```python
from build123d import *

# Parameters (mm, degrees)
SKETCH1_W           = 110
SKETCH1_H           = 30
BOSS_EXTRUDE1_DEPTH = 12
FILLET1_R           = 10
FILLET2_R           = 10
SKETCH9_R           = 12
CUT_EXTRUDE5_DEPTH  = 11
SKETCH13_R          = 12
CUT_EXTRUDE7_DEPTH  = 11
SKETCH15_R          = 3.43
SKETCH15_R_2        = 1
CUT_EXTRUDE8_DEPTH  = 123.394479271
SKETCH16_R          = 3.43
SKETCH16_R_2        = 1
CUT_EXTRUDE9_DEPTH  = 123.394479271


with BuildPart() as part:
    # Sketch1 → Boss-Extrude1 (new body)
    with BuildSketch(Plane(origin=(0, 0, 0), x_dir=(1, 0, 0), z_dir=(0, 1, 0))):
        with Locations((5.385430756, 3.53837453)):
            Rectangle(SKETCH1_W, SKETCH1_H)
    extrude(amount=BOSS_EXTRUDE1_DEPTH)

    # Fillet1
    fillet1_edges = [part.edges().sort_by_distance(p)[0] for p in [
        (-49.614569244, 6, -18.53837453),
        (-49.614569244, 6, 11.46162547),
    ]]
    fillet(fillet1_edges, radius=FILLET1_R)

    # Fillet2
    fillet2_edges = [part.edges().sort_by_distance(p)[0] for p in [
        (60.385430756, 6, -18.53837453),
        (60.385430756, 6, 11.46162547),
    ]]
    fillet(fillet2_edges, radius=FILLET2_R)

    # Sketch9 → Cut-Extrude5 (cut)
    with BuildSketch(Plane(origin=(0, 12, 0), x_dir=(1, 0, 0), z_dir=(0, 1, 0))):
        with Locations(Location((-31.195762423, 3.53837453, 0), (0, 0, 270))):
            Circle(SKETCH9_R)
    extrude(amount=-CUT_EXTRUDE5_DEPTH, mode=Mode.SUBTRACT)

    # Sketch13 → Cut-Extrude7 (cut)
    with BuildSketch(Plane(origin=(70.696833098, 12, 1.072209922), x_dir=(1, 0, 0), z_dir=(0, 1, 0))):
        with Locations(Location((-31.195762423, 3.53837453, 0), (0, 0, 270))):
            Circle(SKETCH13_R)
    extrude(amount=-CUT_EXTRUDE7_DEPTH, mode=Mode.SUBTRACT)

    # Sketch15 → Cut-Extrude8 (cut, through all)
    with BuildSketch(Plane(origin=(70.696833098, 1, 1.072209922), x_dir=(1, 0, 0), z_dir=(0, 1, 0))):
        with Locations(Location((-31.147671482, 3.53837453, 0), (0, 0, 270))):
            Circle(SKETCH15_R)
        with Locations(Location((-25.217671482, 3.53837453, 0), (0, 0, 270))):
            Circle(SKETCH15_R_2)
        with Locations(Location((-37.077671482, 3.53837453, 0), (0, 0, 90))):
            Circle(SKETCH15_R_2)
    extrude(amount=-CUT_EXTRUDE8_DEPTH, mode=Mode.SUBTRACT)

    # Sketch16 → Cut-Extrude9 (cut, through all)
    with BuildSketch(Plane(origin=(70.696833098, 1, 1.072209922), x_dir=(1, 0, 0), z_dir=(0, 1, 0))):
        with Locations(Location((-101.699594536, 4.556727145, 0), (0, 0, 270))):
            Circle(SKETCH16_R)
        with Locations(Location((-95.769594536, 4.556727145, 0), (0, 0, 270))):
            Circle(SKETCH16_R_2)
        with Locations(Location((-107.629594536, 4.556727145, 0), (0, 0, 90))):
            Circle(SKETCH16_R_2)
    extrude(amount=-CUT_EXTRUDE9_DEPTH, mode=Mode.SUBTRACT)


solid = part.part
```
Check sheet for the modelled part. Datum: model origin and axes. Units: mm. A direction names the side the tool comes from. Coordinates: 2 decimals unless noted, no trailing zeros. Write each loop counter-clockwise with the first axis right and the second up, starting at its lowest first coordinate (ties: lowest second). Pieces come first, ordered by that corner, then holes. Notation, with made-up numbers: M -39.5,35 L -18.5,35 A14 cw -18.5,46 Z; hole C 41,5.5 d4. An arc over 180 degrees is marked long. Use one line per item in the form item = value.
Item 1: Sectioned sample at B-B, the plane z = 6.25. Record the cut outline in (x, y), and give its area (3 significant figures).
Answer below:
outline = M -48.39,0 L 59.16,0 L 59.16,12 L 47.75,12 L 47.75,1 L 31.25,1 L 31.25,12 L -24.25,12 L -24.25,1 L -38.14,1 L -38.14,12 L -48.39,12 Z
area = 957 mm^2
Item 2: Set-up check for faces 1 (the face through (42.95, 0.51, -2.91)), 2 (the face through (-19.298, 6.577, -5.101)): record each of +Z, -Z, +X, -X, +Y, -Y from which the full face is reachable in a straight line by a thin tool's end or side.
Answer below:
face_1 = +Y, -Y
face_2 = +Y
Item 3: Sectioned sample at C-C, the plane x = -41. Record the cut outline in (y, z).
Answer below:
outline = M 0,-18.44 L 12,-18.44 L 12,-10.46 L 1,-10.46 L 1,3.38 L 12,3.38 L 12,11.37 L 0,11.37 Z
Item 4: Material ranges on L1, parallel to Z at x = -30.5, y = 3.75; L2, parallel to Z at x = -31, y = 7; L3, parallel to X at y = 8.75, z = -5.5, recorded low to high. Write a range as from..to.
Answer below:
L1 = -18.54..-15.52, 8.44..11.46
L2 = -18.54..-15.54, 8.46..11.46
L3 = -49.61..-43.03, -19.36..27.89, 51.11..60.39
Item 5: Gauge pin test, flat ends, axial feed: pin 1 Ø1.6 at (x, z) = (-36.93, -3.48) entering from -Y; pin 2 Ø7 at (x, z) = (-34, -9) entering from +Y; pin 3 Ø4 at (y, z) = (2, -11) entering from +X. Record the tip position at first contact, or that the pin passes through.
Answer below:
pin_1 = through
pin_2 = 1
pin_3 = 60.37
Item 6: Sectioned sample at A-A, the plane y = 7. Record the cut outline in (x, z).
Answer below:
outline = M -49.61,-8.54 A10 ccw -39.61,-18.54 L 50.39,-18.54 A10 ccw 60.39,-8.54 L 60.39,1.46 A10 ccw 50.39,11.46 L -39.61,11.46 A10 ccw -49.61,1.46 Z; hole C -31.2,-3.54 d24; hole C 39.5,-2.47 d24
Item 7: Sectioned sample at D-D, the plane z = -11.5. Record the cut outline in (x, y), and give its area (3 significant figures).
Answer below:
outline = M -49.17,0 L 59.94,0 L 59.94,12 L 47.4,12 L 47.4,1 L 31.6,1 L 31.6,12 L -22.22,12 L -22.22,1 L -40.17,1 L -40.17,12 L -49.17,12 Z
area = 938 mm^2
